Check sheet for the drawn part. Datum: minimum x, y, z corner. Units: mm. Round coordinates to 2 decimals unless told otherwise and drop trailing zeros. Write each loop counter-clockwise with the first axis right and the second up, starting at its lowest first coordinate (ties: lowest second). Pieces come first, ordered by that corner, then holes. Notation, with made-up numbers: (81, 55.25) -> (111, 55.25) arc R8 ccw to (111, 70.25) -> close; hole circle Ø4 at (87.25, 66). An arc over 180 degrees is marked (long way). Use a Markdown table: item, result.
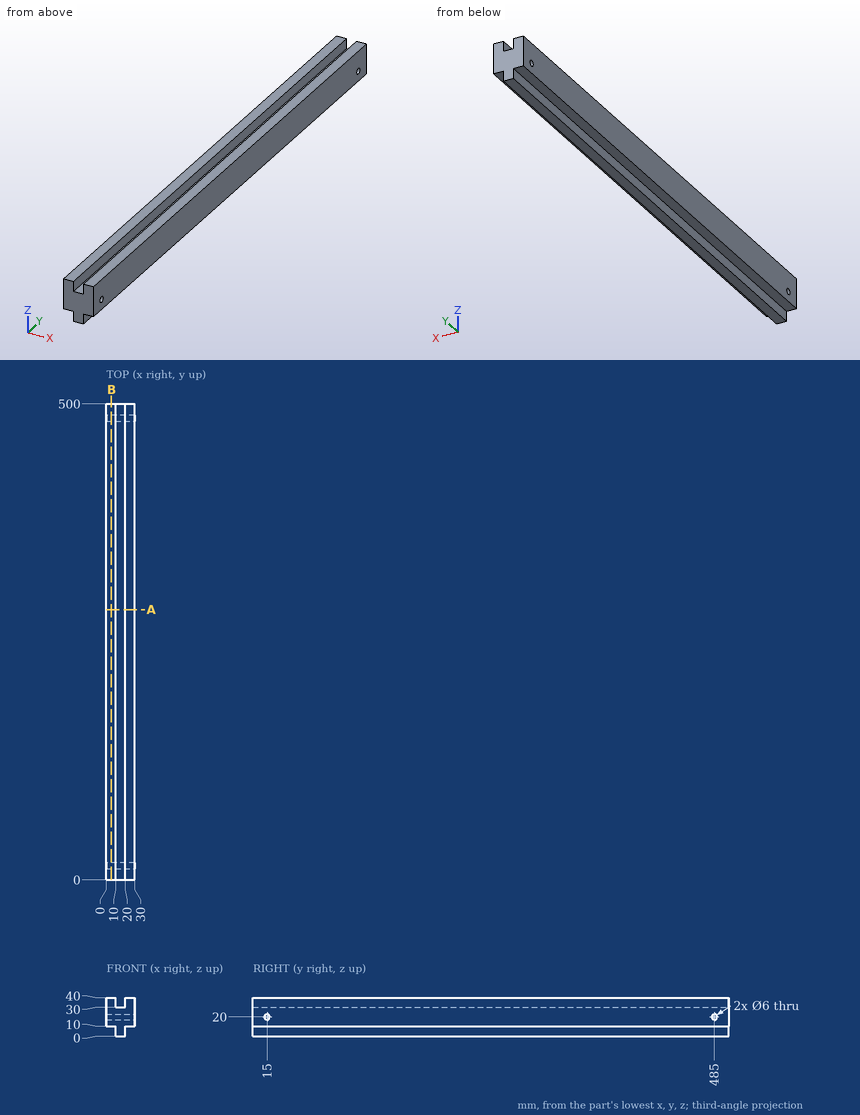
(1) Section check A-A on y = 284. Record the cut outline in (x, z).
A:
| item | result |
|---|---|
| outline | (0, 10) -> (10, 10) -> (10, 0) -> (20, 0) -> (20, 10) -> (30, 10) -> (30, 40) -> (20, 40) -> (20, 30) -> (10, 30) -> (10, 40) -> (0, 40) -> close |
(2) Thickness scan on line 1 (X direction, y = 322, z = 38.5); line 2 (Z direction, x = 17, y = 485); line 3 (Y direction, x = 25.5, z = 18). Record the ranges inside material, lowest first.
A:
| item | result |
|---|---|
| line 1 | x = 0 to 10, 20 to 30 |
| line 2 | z = 0 to 17, 23 to 30 |
| line 3 | y = 0 to 12.76, 17.24 to 482.76, 487.24 to 500 |
(3) Gauge pin test, flat ends, axial feed: pin 1 Ø5 at (y, z) = (277, 37) entering from -X; pin 2 Ø3 at (x, y) = (13, 159) entering from +Z; pin 3 Ø5 at (x, y) = (4.5, 362) entering from -Z; pin 4 Ø2 at (y, z) = (294, 6.5) entering from +X. Record the tip position at first contact, or that the pin passes through.
A:
| item | result |
|---|---|
| pin 1 | stops at x = 0 |
| pin 2 | stops at z = 30 |
| pin 3 | stops at z = 10 |
| pin 4 | stops at x = 20 |
(4) Section check B-B on x = 5.25. Record the cut outline in (y, z), plus the area to 3 significant figures.
A:
| item | result |
|---|---|
| outline | (0, 10) -> (500, 10) -> (500, 40) -> (0, 40) -> close; hole circle Ø6 at (15, 20); hole circle Ø6 at (485, 20) |
| area | 14,900 mm2 |
